```python
from build123d import *

# Parameters (mm, degrees)
SWEEP_THIN1_PROFILE_R   = 145
SWEEP_THIN1_PROFILE_R_2 = 105
BOSS_EXTRUDE1_START     = -50
SKETCH16_R              = 15
SKETCH16_R_2            = 145
BOSS_EXTRUDE1_DEPTH     = 50
SKETCH17_R              = 30
CUT_EXTRUDE1_DEPTH      = 10
CIRPATTERN1_COUNT       = 2
CIRPATTERN1_ANGLE       = 90
CHAMFER1_SIZE           = 10
FILLET1_R               = 10
CUT_EXTRUDE3_DEPTH      = 10
CIRPATTERN4_COUNT       = 2
CIRPATTERN4_ANGLE       = 90


with BuildPart() as part:
    # Sweep-Thin1: sweep along a path in Sketch1
    with BuildLine(Plane.XY) as sweep_thin1_path:
        Line((0, 410), (0, 260))
        ThreePointArc((0, 260), (76.152236891, 76.152236891), (260, 0))
        Line((260, 0), (410, 0))
    # Sweep-Thin1 profile (on start of the path) → Sweep-Thin1 (sweep)
    with BuildSketch(Plane(origin=(0, 410, 0), x_dir=(-1, 0, 0), z_dir=(0, -1, 0))):
        Circle(SWEEP_THIN1_PROFILE_R)
        Circle(SWEEP_THIN1_PROFILE_R_2, mode=Mode.SUBTRACT)
    sweep(path=sweep_thin1_path.line)

    # Sketch16 → Boss-Extrude1 (add)
    with BuildSketch(Plane(origin=(0, 410, 0), x_dir=(1, 0, 0), z_dir=(0, 1, 0)).offset(BOSS_EXTRUDE1_START)):
        with BuildLine():
            Line((-160, 180), (160, 180))
            ThreePointArc((160, 180), (174.142135624, 174.142135624), (180, 160))
            Line((180, 160), (180, -160))
            ThreePointArc((180, -160), (174.142135624, -174.142135624), (160, -180))
            Line((160, -180), (-160, -180))
            ThreePointArc((-160, -180), (-174.142135624, -174.142135624), (-180, -160))
            Line((-180, -160), (-180, 160))
            ThreePointArc((-180, 160), (-174.142135624, 174.142135624), (-160, 180))
        make_face()
        with Locations(Location((-130, -130, 0), (0, 0, 180))):
            Circle(SKETCH16_R, mode=Mode.SUBTRACT)
        with Locations(Location((130, -130, 0), (0, 0, 180))):
            Circle(SKETCH16_R, mode=Mode.SUBTRACT)
        with Locations(Location((-130, 130, 0), (0, 0, 180))):
            Circle(SKETCH16_R, mode=Mode.SUBTRACT)
        with Locations(Location((130, 130, 0), (0, 0, 180))):
            Circle(SKETCH16_R, mode=Mode.SUBTRACT)
        with Locations(Location((0, 0, 0), (0, 0, 180))):
            Circle(SKETCH16_R_2, mode=Mode.SUBTRACT)
    boss_extrude1 = extrude(amount=BOSS_EXTRUDE1_DEPTH)

    # Sketch17 → Cut-Extrude1 (cut)
    with BuildSketch(Plane(origin=(0, 410, 0), x_dir=(1, 0, 0), z_dir=(0, 1, 0))):
        with Locations(Location((-130, 130, 0), (0, 0, 180))):
            Circle(SKETCH17_R)
        with Locations(Location((130, 130, 0), (0, 0, 180))):
            Circle(SKETCH17_R)
        with Locations(Location((130, -130, 0), (0, 0, 180))):
            Circle(SKETCH17_R)
        with Locations(Location((-130, -130, 0), (0, 0, 180))):
            Circle(SKETCH17_R)
    cut_extrude1 = extrude(amount=-CUT_EXTRUDE1_DEPTH, mode=Mode.SUBTRACT)

    # CirPattern1: Boss-Extrude1, Cut-Extrude1 ×2 about axis
    cirpattern1_axis = Axis((0, 0, 0), (0, 0, -1))
    add([boss_extrude1.rotate(cirpattern1_axis, i * CIRPATTERN1_ANGLE / (CIRPATTERN1_COUNT - 1)) for i in range(1, CIRPATTERN1_COUNT)])
    add([cut_extrude1.rotate(cirpattern1_axis, i * CIRPATTERN1_ANGLE / (CIRPATTERN1_COUNT - 1)) for i in range(1, CIRPATTERN1_COUNT)], mode=Mode.SUBTRACT)

    # Chamfer1
    chamfer1_edges = [part.edges().sort_by_distance(p)[0] for p in [
        (105, 410, 0),
        (410, 105, 0),
    ]]
    chamfer(chamfer1_edges, length=CHAMFER1_SIZE)

    # Fillet1
    fillet1_edges = [part.edges().sort_by_distance(p)[0] for p in [
        (145, 360, 0),
        (360, 145, 0),
    ]]
    fillet(fillet1_edges, radius=FILLET1_R)

    # Sketch25 → Cut-Extrude3 (cut)
    with BuildSketch(Plane.XZ.offset(-360)):
        Polygon((-104.019237886, -130), (-117.009618943, -107.5), (-142.990381057, -107.5), (-155.980762114, -130), (-142.990381057, -152.5), (-117.009618943, -152.5), align=None)
        Polygon((104.019237886, 130), (117.009618943, 107.5), (142.990381057, 107.5), (155.980762114, 130), (142.990381057, 152.5), (117.009618943, 152.5), align=None)
        Polygon((117.009618943, -107.5), (104.019237886, -130), (117.009618943, -152.5), (142.990381057, -152.5), (155.980762114, -130), (142.990381057, -107.5), align=None)
        Polygon((-142.990381057, 152.5), (-155.980762114, 130), (-142.990381057, 107.5), (-117.009618943, 107.5), (-104.019237886, 130), (-117.009618943, 152.5), align=None)
    cut_extrude3 = extrude(amount=-CUT_EXTRUDE3_DEPTH, mode=Mode.SUBTRACT)

    # CirPattern4: Cut-Extrude3 ×2 about axis
    cirpattern4_axis = Axis((0, 0, 0), (0, 0, -1))
    for i in range(1, CIRPATTERN4_COUNT):
        add(cut_extrude3.rotate(cirpattern4_axis, i * CIRPATTERN4_ANGLE / (CIRPATTERN4_COUNT - 1)), mode=Mode.SUBTRACT)


solid = part.part
```
Can you work these out from the model? Positions are in its coordinate system, mm. A direction names the side the tool comes from. Coordinates: 2 decimals unless noted, no trailing zeros. Answer as a JSON object with one key per item and string values.
1) For faces 5 (the face through (136.503, 405.07, -159.287)), 6 (the face through (-118.8, 370, 140.3)), 7 (the face through (370, 118.8, 140.3)), which set-ups out of +Z, -Z, +X, -X, +Y, -Y let a thin tool reach every point of the face, with its end or its side?
Results:
{"face 5": "+Y", "face 6": "-Y", "face 7": "none"}
2) For P1, Ø8, axis at x = 310, z = -79, coming from the -Y side; P2, Ø2, axis at y = 339.5, z = 39, coming from the -X side; P3, Ø10, axis at y = 248, z = -118.5, coming from the +X side, each with a flat end and sliding along its axis, tell me the tip position at first contact or that it passes through.
Results:
{"P1": "stops at y = -124.1", "P2": "stops at x = -139.93", "P3": "stops at x = 90.67"}
3) Imagine slicing it at B-B (x = 130). Count the separate pieces of the cut face and the enclosed holes in it, then the cut area to 3 significant figures.
Results:
{"separate pieces": "3", "enclosed holes": "1", "area": "71,400 mm^2"}
4) If I drill on line 1 (Z direction, x = 402, y = 130); line 2 (Z direction, x = -130, y = 391), over which ranges is the centre line in solid material (lowest first)?
Results:
{"line 1": "z = -180 to -160, -100 to 100, 160 to 180", "line 2": "z = -180 to -145, -115 to 115, 145 to 180"}
5) Thinking about a two-plate mould opening in Z: for faces 1 (the face through (410, -83, -83)), 2 (the face through (384.65, 173.986, 174.297)), 3 (the face through (124, 400, 144)), 4 (the face through (141.2, 370, -119.7)), which applies, pulls with the +Z half, pulls with the -Z half, needs draft (parallel to the pull), parting line crosses it, or undercut?
Results:
{"face 1": "needs draft", "face 2": "pulls with the +Z half", "face 3": "undercut", "face 4": "undercut"}
